from build123d import *

# Parameters (mm, degrees)
F1_DEPTH = 30
F3_DEPTH = 30
F4_R     = 10
F5_DEPTH = 25


with BuildPart() as f1:
    # F0 (on Front) → F1 (new body, symmetric)
    with BuildSketch(Plane.XZ):
        Polygon((0, 40), (-20, 40), (-20, 0), (20, 0), (20, 20), align=None)
    extrude(amount=F1_DEPTH, both=True)

    # F2 (on face) → F3 (cut)
    with BuildSketch(Plane.XY.offset(40)):
        Polygon((10, 20), (-20, 20), (-20, -20), (10, -20), (10, -10), (20, -10), (20, 10), (10, 10), align=None)
    extrude(amount=-F3_DEPTH, mode=Mode.SUBTRACT)

    # F4 (on face) → F5 (cut)
    with BuildSketch(Plane.XY.offset(10)):
        Circle(F4_R)
    extrude(amount=-F5_DEPTH, mode=Mode.SUBTRACT)


solid = f1.part
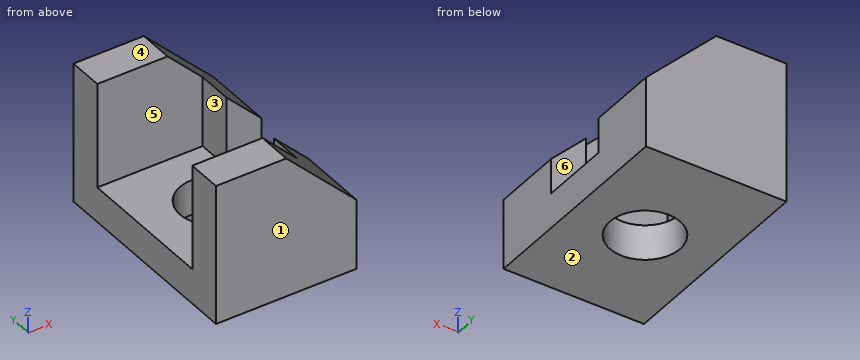
The listing builds one solid part. Answer for the finished solid, in the listing's coordinates (mm). Face numbers are marked on the shaded views. A direction names the side the tool comes from. Give positions to 0.01 mm unless a question says otherwise; leave off trailing zeros. Write each loop counter-clockwise with the first axis right and the second up, starting at its lowest first coordinate (ties: lowest second). Pieces come first, ordered by that corner, then holes. Notation, with made-up numbers: (75.25, 35.25) - (114.25, 35.25) arc R16 cw to (114.25, 43.25) - close; hole circle Ø3 at (81.25, 20.5). An arc over 180 degrees is marked (long way). Use a Markdown table: item, result.
1. Section D-D on x = 12 is taken. Write down the section's boundary in (y, z), plus the area to 3 significant figures.
Values follow:
| item | result |
|---|---|
| outline | (-30, 0) - (30, 0) - (30, 28) - (10, 28) - (10, 10) - (-10, 10) - (-10, 28) - (-30, 28) - close |
| area | 1,320 mm² |
2. Find the intervals of material crossed by probe 1 along Y at (x, z) = (0, 4); probe 2 along Y at (x, z) = (-4, 27.5); probe 3 along Z at (x, y) = (-11.5, -10.5), in increasing order. Write a range as from..to.
Values follow:
| item | result |
|---|---|
| probe 1 | y = -30..-10, 10..30 |
| probe 2 | y = -30..-20, 20..30 |
| probe 3 | z = 0..10 |
3. Section A-A on z = 27.5 is taken. Write down the section's boundary in (x, y).
Values follow:
| item | result |
|---|---|
| outline | (-20, -30) - (12.5, -30) - (12.5, -10) - (10, -10) - (10, -20) - (-20, -20) - close; (-20, 20) - (10, 20) - (10, 10) - (12.5, 10) - (12.5, 30) - (-20, 30) - close |
4. A tool of negligible diameter and unlimited length cuts with its end or side. For the marked faces 4, 5 and 6, from which of +Z, -Z, +X, -X, +Y, -Y can it reach the whole face along a straight path? Write none if from no direction.
Values follow:
| item | result |
|---|---|
| face 4 | +Z, +X, -X, +Y, -Y |
| face 5 | +Z, -X |
| face 6 | +Z, +X, -X |
5. For a pull along Y with two mould halves and no side action, classify the marked faces 1, 2 and 3 as released by +Y, released by -Y, zero draft, split by the parting line, or undercut.
Values follow:
| item | result |
|---|---|
| face 1 | released by -Y |
| face 2 | zero draft |
| face 3 | undercut |
6. Section C-C on x = 6 is taken. Write down the section's boundary in (y, z).
Values follow:
| item | result |
|---|---|
| outline | (-30, 0) - (-8, 0) - (-8, 10) - (-20, 10) - (-20, 34) - (-30, 34) - close; (8, 0) - (30, 0) - (30, 34) - (20, 34) - (20, 10) - (8, 10) - close |
7. Section B-B on y = 0 is taken. Write down the section's boundary in (x, z), plus the area to 3 significant figures.
Values follow:
| item | result |
|---|---|
| outline | (-20, 0) - (-10, 0) - (-10, 10) - (-20, 10) - close; (10, 0) - (20, 0) - (20, 10) - (10, 10) - close |
| area | 200 mm² |
8. Each of these flat-tipped pins is pushed along its axis until it touches: P1, Ø16, axis at x = 0, y = 0, coming from the +Z side; P2, Ø2, axis at y = -12, z = 24, coming from the -X side. Where does it stop, or does it pass through?
Values follow:
| item | result |
|---|---|
| P1 | passes through |
| P2 | stops at x = 10 |
